The model under review builds one solid part; all positions refer to its coordinate system, in mm. A direction names the side the tool comes from. Coordinates: 2 decimals unless noted, no trailing zeros. Write each loop counter-clockwise with the first axis right and the second up, starting at its lowest first coordinate (ties: lowest second). Pieces come first, ordered by that corner, then holes. Notation, with made-up numbers: (-36.5, 5.25) - (12.5, 5.25) arc R31 cw to (12.5, 42.25) - close; hole circle Ø11 at (48, -36.75). An arc over 180 degrees is marked (long way). Put each result on its own line as item: value.
Autodesk Fusion 360 part; units mm, degrees
sketch "Sketch1" plane through (0, 0, 0) normal (0, 0, 1) x (1, 0, 0)
  circle A0 centre (0, 0) radius 4
extrude "Extrude1" add sketch "Sketch1" along normal blind 14
sketch "Sketch2" plane through (0, 0, 14) normal (0, 0, 1) x (-1, 0, 0)
  circle A0 centre (0, 0) radius 4
  circle A1 centre (0, 0) radius 6
extrude "Extrude2" add sketch "Sketch2" against normal blind 4
chamfer "Chamfer1" distance 0.5 angle 45 1 edges at (5.594, 2.1697, 14)
chamfer "Chamfer2" distance 0.5 angle 45 1 edges at (-3.7293, -1.4465, 0)
sketch "Sketch3" plane through (0, 0, 14) normal (0, 0, 1) x (-1, 0, 0)
  circle A0 centre (0, 0) radius 5.5
  line L0 (2, -1.1547) -> (2, 1.1547)
  line L1 (-2, 1.1547) -> (-2, -1.1547)
  line L2 (2, -1.1547) -> (0, -2.3094)
  line L3 (0, -2.3094) -> (-2, -1.1547)
  line L4 (2, 1.1547) -> (0, 2.3094)
  line L5 (-2, 1.1547) -> (0, 2.3094)
extrude "Extrude3" cut sketch "Sketch3" against normal blind 4 contours L0 L1 L2 L3 L4 L5
1. Consider section B-B on y = 0. State the section outline as (x, z) points, plus the area to 4 significant figures.
Determined:
outline: (-6, 10) - (-4, 10) - (-4, 0.5) - (-3.5, 0) - (3.5, 0) - (4, 0.5) - (4, 10) - (6, 10) - (6, 13.5) - (5.5, 14) - (2, 14) - (2, 10) - (-2, 10) - (-2, 14) - (-5.5, 14) - (-6, 13.5) - close
area: 111.5 mm^2
2. To check wall thickness, follow probe 1 along Z at (x, y) = (5, -1.5); probe 2 along Z at (x, y) = (-0.25, 0.5); probe 3 along Y at (x, z) = (0, 1). State the ranges of each line that lie inside material, in increasing order.
Determined:
probe 1: z = 10 to 14
probe 2: z = 0 to 10
probe 3: y = -4 to 4
3. Consider section A-A on z = 13.25. State the section outline as (x, y) points, plus the area to 3 significant figures.
Determined:
outline: circle Ø12 at (0, 0); hole (-2, -1.15) - (0, -2.31) - (2, -1.15) - (2, 1.15) - (0, 2.31) - (-2, 1.15) - close
area: 99.2 mm^2
4. The part is to be moulded in two halves that separate along Y. For faces 3 (the flat face through (2, 0, 12)), 4 (the cylindrical face through (-0.867, 3.905, 5.184)), 5 (the flat face through (0, 0, 10)), 6 (the flat face through (1.42, 3.92, 10)), say which applies: +Y half, -Y half, draft (parallel to the pull), parting line (faces both ways), or undercut.
Determined:
face 3: undercut
face 4: parting line
face 5: undercut
face 6: draft
5. Consider section C-C on z = 3.5. State the section outline as (x, y) points.
Determined:
outline: circle Ø8 at (0, 0)
6. For pin 1 Ø1.5 at (y, z) = (-2, 3.5) entering from -X; pin 2 Ø3 at (y, z) = (-0.5, 5) entering from -X; pin 3 Ø1.5 at (x, z) = (-1.5, 6) entering from -Y, all flat-tipped, find the tip position at first contact; note any pin that passes through.
Determined:
pin 1: stops at x = -3.8
pin 2: stops at x = -4
pin 3: stops at y = -3.93
7. Machinability: for faces 1 (the flat face through (-2.4, -0.1, 14)), 2 (the flat face through (-1.014, -1.724, 12.028)), which of the approach directions +Z, -Z, +X, -X, +Y, -Y give a long, thin tool a straight path to every point of the face, cutting with its end or side? Answer none if there is none.
Determined:
face 1: +Z, +X, -X, +Y, -Y
face 2: +Z
